```python
from build123d import *

# Parameters (mm, degrees)
SKETCH1_R               = 25
BOSS_EXTRUDE1_DEPTH     = 17.5
SKETCH4_R               = 30
BOSS_EXTRUDE2_DEPTH     = 25
CUT_EXTRUDE1_DEPTH      = 165.696691051
CUT_EXTRUDE1_DEPTH_BACK = 165.696691051
SKETCH6_W               = 34
SKETCH6_H               = 34
CUT_EXTRUDE2_DEPTH      = 7
SKETCH7_R               = 3.9
BOSS_EXTRUDE3_DEPTH     = 7
BOSS_EXTRUDE3_TAPER     = 2
CUT_EXTRUDE3_START      = -30
SKETCH8_W               = 42
SKETCH8_H               = 22
CUT_EXTRUDE3_DEPTH      = 30


with BuildPart() as part:
    # Sketch1 → Boss-Extrude1 (new, symmetric)
    with BuildSketch(Plane.XY):
        Circle(SKETCH1_R)
    extrude(amount=BOSS_EXTRUDE1_DEPTH, both=True)

    # Loft1: read off the stored shape, not the designer's step
    # Loft1: loft between two sections, ruled curve by curve
    loft1_from = [
        Edge.make_bspline([(0, 9.43003665, -11.665093603), (0, 32.760223857, 7.194979697), (0, 13.900150557, 30.525166904), (0, -9.43003665, 11.665093603), (0, -32.760223857, -7.194979697), (0, -13.900150557, -30.525166904), (0, 9.43003665, -11.665093603)], [0, 0, 0, 0, 0.5, 0.5, 0.5, 1, 1, 1, 1], 3, [1, 0.333333333, 0.333333333, 1, 0.333333333, 0.333333333, 1]),
    ]
    loft1_to = [
        Edge.make_bspline([(130, 5.054457016, -14.122764045), (130, 33.299985106, -4.013850014), (130, 23.191071075, 24.231678077), (130, -5.054457016, 14.122764045), (130, -33.299985106, 4.013850014), (130, -23.191071075, -24.231678077), (130, 5.054457016, -14.122764045)], [0, 0, 0, 0, 0.5, 0.5, 0.5, 1, 1, 1, 1], 3, [1, 0.333333333, 0.333333333, 1, 0.333333333, 0.333333333, 1]),
    ]
    loft1 = Solid(Shell([*[Face.make_surface_from_curves(loft1_from[k], loft1_to[k]) for k in range(1)], Face(Wire(loft1_from)), Face(Wire(loft1_to))]))
    add(loft1)

    # Sketch4 → Boss-Extrude2 (add, symmetric)
    with BuildSketch(Plane.XY):
        with Locations((130, 0)):
            Circle(SKETCH4_R)
    extrude(amount=BOSS_EXTRUDE2_DEPTH, both=True)

    # Sketch5 → Cut-Extrude1 (cut, two sides: drawn at the far end of the back side and taken through both)
    with BuildSketch(Plane(origin=(0, 0, 0), x_dir=(1, 0, 0), z_dir=(0, 1, 0)).offset(-CUT_EXTRUDE1_DEPTH_BACK)):
        with BuildLine():
            Line((35, 7), (85, 7))
            ThreePointArc((85, 7), (92, 0), (85, -7))
            Line((85, -7), (35, -7))
            ThreePointArc((35, -7), (28, 0), (35, 7))
        make_face()
    extrude(amount=CUT_EXTRUDE1_DEPTH + CUT_EXTRUDE1_DEPTH_BACK, mode=Mode.SUBTRACT)

    # Sketch6 → Cut-Extrude2 (cut)
    with BuildSketch(Plane.XY.offset(17.5)):
        Rectangle(SKETCH6_W, SKETCH6_H)
    extrude(amount=-CUT_EXTRUDE2_DEPTH, mode=Mode.SUBTRACT)

    # Sketch7 → Boss-Extrude3 (add)
    with BuildSketch(Plane(origin=(0, 0, -17.5), x_dir=(-1, 0, 0), z_dir=(0, 0, -1))):
        Circle(SKETCH7_R)
    extrude(amount=BOSS_EXTRUDE3_DEPTH, taper=BOSS_EXTRUDE3_TAPER)

    # Sketch8 → Cut-Extrude3 (cut)
    with BuildSketch(Plane(origin=(0, 0, -25), x_dir=(-1, 0, 0), z_dir=(0, 0, -1)).offset(CUT_EXTRUDE3_START)):
        with Locations((-134, 0)):
            Rectangle(SKETCH8_W, SKETCH8_H)
        with BuildLine():
            Line((-165, -6), (-159.393876913, -6))
            ThreePointArc((-159.393876913, -6), (-160, 0), (-159.393876913, 6))
            Line((-159.393876913, 6), (-165, 6))
            Line((-165, 6), (-165, -6))
        make_face()
        with BuildLine():
            Line((-159.393876913, -6), (-155, -6))
            Line((-155, -6), (-155, 6))
            Line((-155, 6), (-159.393876913, 6))
            ThreePointArc((-159.393876913, 6), (-160, 0), (-159.393876913, -6))
        make_face()
    extrude(amount=CUT_EXTRUDE3_DEPTH, mode=Mode.SUBTRACT)


solid = part.part
```
Could you check a few things on this model? Use its own coordinates, in mm. A direction names the side the tool comes from. Give positions to 0.01 mm unless a question says otherwise; leave off trailing zeros. Order: outer loops, then holes, each group sorted by start corner. A loop starts at its lowest first (then second) coordinate and runs counter-clockwise, first axis right, second up.
Q1. Suppose I cut it at A-A, the plane x = 0. Write out the boundary of the cut face in (y, z).
Q2. If I drill on line 1 along X through (y, z) = (-9, -17); line 2 along X through (y, z) = (-13, 14); line 3 along X through (y, z) = (-1.5, -22), over which ranges is the centre line in solid material (lowest first)?
Q3. For faces 1 (the flat face through (60, 0, -7)), 2 (the flat face through (0, 0, 10.5)), 3 (the flat face through (157, 6, -10)), 4 (the flat face through (0, 0, -24.5)), which set-ups out of +Z, -Z, +X, -X, +Y, -Y let a thin tool reach every point of the face, with its end or its side?
Q4. I'm going to push flat-ended pins straight in: P1, Ø10, axis at y = -9, z = 19.5, coming from the +X side; P2, Ø1.3, axis at x = 156.5, z = -14, coming from the -Y side; P3, Ø21, axis at x = 62.5, y = -3.5, coming from the +Z side. Where does each tip first touch, or does it pass through?
Q5. We'd pull the mould along X, two halves only. Please class faces 5 (the flat face through (2, -18, 17.5)), 6 (the cylindrical face through (158.615, 9.011, 0.35)): +X half, -X half, draft (parallel to the pull), parting line (faces both ways), or undercut.
Q6. Suppose I cut it at B-B, the plane z = 22.5. Write out the boundary of the cut face in (x, y).
Q7. Suppose I cut it at C-C, the plane x = 130. Write out the boundary of the cut face in (y, z), and give its area (3 significant figures).
Solution:
1. outline: (-25, -17.5) - (-3.9, -17.5) - (-3.66, -24.5) - (3.66, -24.5) - (3.9, -17.5) - (25, -17.5) - (25, 17.5) - (17, 17.5) - (17, 10.5) - (-17, 10.5) - (-17, 17.5) - (-25, 17.5) - close
2. line 1: x = -23.32 to 23.32, 101.38 to 113, 155 to 158.62
2. line 2: x = -21.35 to -17, 17 to 21.35, 102.96 to 157.04
2. line 3: x = -3.43 to 3.43, 100.04 to 113
3. face 1: +Y, -Y
3. face 2: +Z
3. face 3: -Z, +X
3. face 4: -Z, -X, +Y, -Y
4. P1: stops at x = 159.73
4. P2: stops at y = -15.22
4. P3: stops at z = 14.8
5. face 5: draft
5. face 6: undercut
6. outline: circle Ø60 at (130, 0)
7. outline: (-30, -25) - (-11, -25) - (-11, 5) - (11, 5) - (11, -25) - (30, -25) - (30, 25) - (-30, 25) - close
7. area: 2,340 mm2
